Study the drawing (mm; zero at the part's minimum x, y, z) and answer. A direction names the side the tool comes from. Coordinates: 2 decimals unless noted, no trailing zeros. Order: outer loops, then holes, each group sorted by start corner. A loop starts at its lowest first (then second) coordinate and runs counter-clockwise, first axis right, second up.
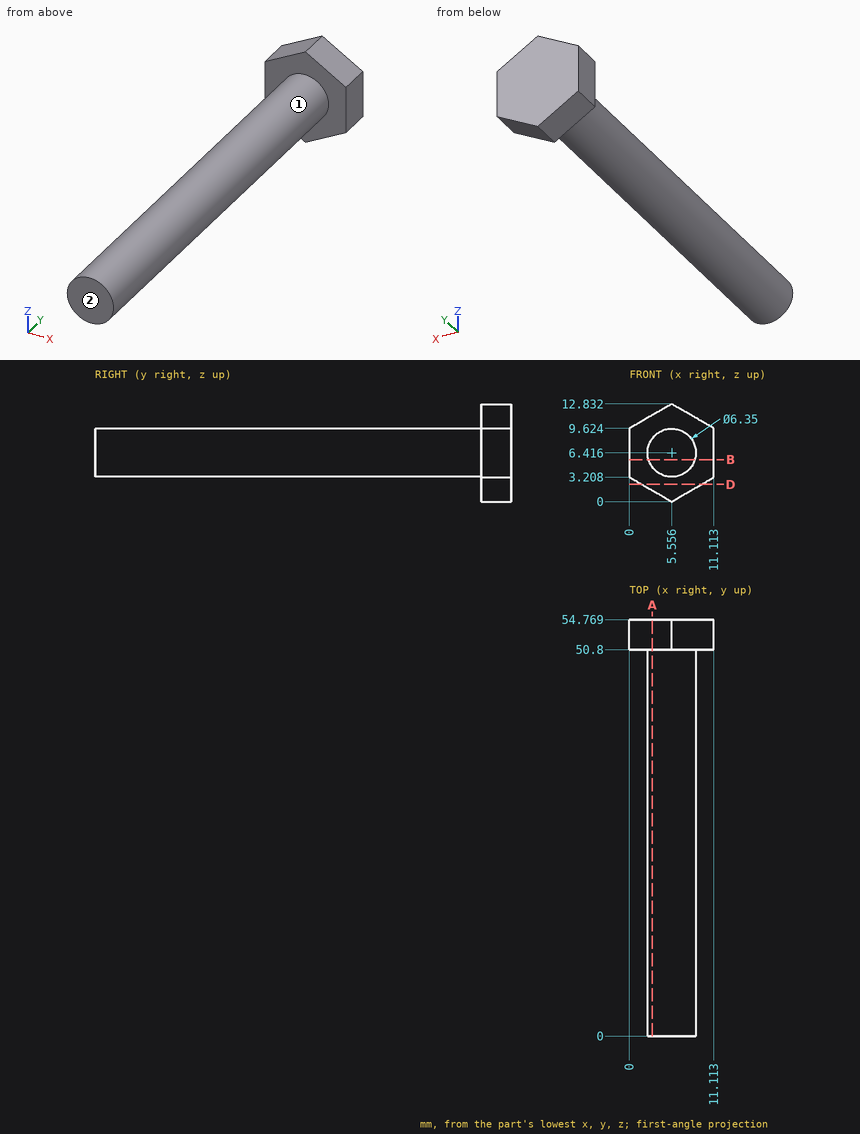
(1) For the marked faces 1 and 2, determine the directions among +Z, -Z, +X, -X, +Y, -Y from which every point of the face is accessible in a straight line to the end or side of a thin tool.
(2) Each of these flat-tipped pins is pushed along its axis until it touches: pin 1 Ø6 at (x, y) = (1.5, 7) entering from -Z; pin 2 Ø6 at (x, y) = (2.5, 21) entering from +Z; pin 3 Ø3.5 at (x, z) = (3.5, 8) entering from -Y. Where does it stop, or does it pass through?
(3) Consider line 1 (Y direction, x = 9.75, z = 2.5); line 2 (X direction, y = 45, z = 6.5); line 3 (Z direction, x = 5.5, y = 19). Determine where each line is inside the solid, lowest interval first.
(4) Find section D-D (z = 2.25). Write down the section's boundary in (x, y).
(5) Find section A-A (x = 3). Write down the section's boundary in (y, z) (1 decimal).
(6) Find section B-B (z = 5.5). Write down the section's boundary in (x, y), and give its area (3 significant figures).
Findings below:
1. face 1: -Y
1. face 2: +Z, -Z, +X, -X, -Y
2. pin 1: stops at z = 3.42
2. pin 2: stops at z = 9.59
2. pin 3: stops at y = 0
3. line 1: y = 50.8 to 54.77
3. line 2: x = 2.38 to 8.73
3. line 3: z = 3.24 to 9.59
4. outline: (1.66, 50.8) - (9.45, 50.8) - (9.45, 54.77) - (1.66, 54.77) - close
5. outline: (0, 4.5) - (50.8, 4.5) - (50.8, 1.5) - (54.8, 1.5) - (54.8, 11.4) - (50.8, 11.4) - (50.8, 8.3) - (0, 8.3) - close
6. outline: (0, 50.8) - (2.52, 50.8) - (2.52, 0) - (8.6, 0) - (8.6, 50.8) - (11.11, 50.8) - (11.11, 54.77) - (0, 54.77) - close
6. area: 353 mm2
